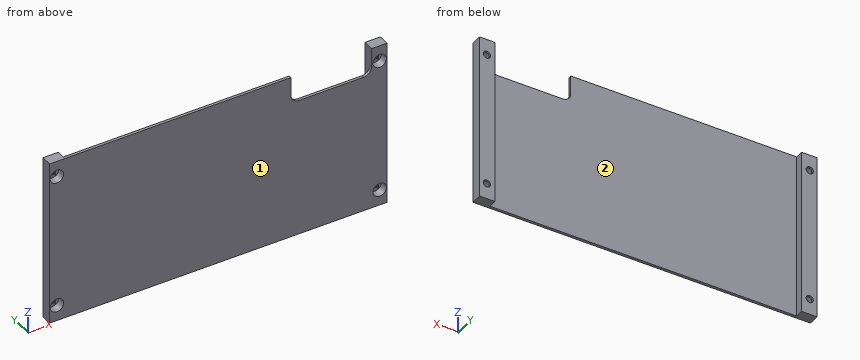
```python
from build123d import *

# Parameters (mm, degrees)
SKETCH1_W           = 126
SKETCH1_H           = 61.8
BOSS_EXTRUDE1_DEPTH = 1
SKETCH2_W           = 6
SKETCH2_H           = 61.8
BOSS_EXTRUDE2_DEPTH = 3
SKETCH3_R           = 1.35
CUT_EXTRUDE1_DEPTH  = 5
SKETCH4_R           = 2.5
CUT_EXTRUDE2_DEPTH  = 3
SKETCH5_W           = 30
SKETCH5_H           = 10
CUT_EXTRUDE3_DEPTH  = 5
FILLET1_R           = 3
CUT_EXTRUDE4_DEPTH  = 0.2
SKETCH7_W           = 2.7
SKETCH7_H           = 2.7
CUT_EXTRUDE5_DEPTH  = 0.2
SKETCH8_W           = 0.3
SKETCH8_H           = 61.8
CUT_EXTRUDE6_DEPTH  = 5


with BuildPart() as part:
    # Sketch1 → Boss-Extrude1 (new body)
    with BuildSketch(Plane(origin=(0, 0, 0), x_dir=(1, 0, 0), z_dir=(0, 1, 0))):
        Rectangle(SKETCH1_W, SKETCH1_H)
    extrude(amount=BOSS_EXTRUDE1_DEPTH)

    # Sketch2 → Boss-Extrude2 (add)
    with BuildSketch(Plane(origin=(0, 1, 0), x_dir=(1, 0, 0), z_dir=(0, 1, 0))):
        with Locations((-60, 0)):
            Rectangle(SKETCH2_W, SKETCH2_H)
        with Locations((60, 0)):
            Rectangle(SKETCH2_W, SKETCH2_H)
    extrude(amount=BOSS_EXTRUDE2_DEPTH)

    # Sketch3 → Cut-Extrude1 (cut, through all)
    with BuildSketch(Plane(origin=(0, 4, 0), x_dir=(1, 0, 0), z_dir=(0, 1, 0))):
        with Locations((-60, 25)):
            Circle(SKETCH3_R)
        with Locations((-60, -25)):
            Circle(SKETCH3_R)
        with Locations((60, -25)):
            Circle(SKETCH3_R)
        with Locations((60, 25)):
            Circle(SKETCH3_R)
    extrude(amount=-CUT_EXTRUDE1_DEPTH, mode=Mode.SUBTRACT)

    # Sketch4 → Cut-Extrude2 (cut)
    with BuildSketch(Plane.XZ):
        with Locations((60, -25)):
            Circle(SKETCH4_R)
        with Locations((60, 25)):
            Circle(SKETCH4_R)
        with Locations((-60, 25)):
            Circle(SKETCH4_R)
        with Locations((-60, -25)):
            Circle(SKETCH4_R)
    extrude(amount=-CUT_EXTRUDE2_DEPTH, mode=Mode.SUBTRACT)

    # Sketch5 → Cut-Extrude3 (cut, through all)
    with BuildSketch(Plane.XZ):
        with Locations((42, 25.9)):
            Rectangle(SKETCH5_W, SKETCH5_H)
    extrude(amount=-CUT_EXTRUDE3_DEPTH, mode=Mode.SUBTRACT)

    # Fillet1
    fillet1_edges = [part.edges().sort_by_distance(p)[0] for p in [
        (27, 0.5, 20.9),
        (57, 0.5, 20.9),
    ]]
    fillet(fillet1_edges, radius=FILLET1_R)

    # Sketch6 → Cut-Extrude4 (cut)
    with BuildSketch(Plane.XZ.offset(-3)):
        with BuildLine():
            Line((-61.35, 22.895837459), (-61.35, 27.104162541))
            ThreePointArc((-61.35, 27.104162541), (-60, 27.5), (-58.65, 27.104162541))
            Line((-58.65, 27.104162541), (-58.65, 22.895837459))
            ThreePointArc((-58.65, 22.895837459), (-60, 22.5), (-61.35, 22.895837459))
        make_face()
        with BuildLine():
            Line((-61.35, -27.104162541), (-61.35, -22.895837459))
            ThreePointArc((-61.35, -22.895837459), (-60, -22.5), (-58.65, -22.895837459))
            Line((-58.65, -22.895837459), (-58.65, -27.104162541))
            ThreePointArc((-58.65, -27.104162541), (-60, -27.5), (-61.35, -27.104162541))
        make_face()
    cut_extrude4 = extrude(amount=-CUT_EXTRUDE4_DEPTH, mode=Mode.SUBTRACT)

    # Sketch7 → Cut-Extrude5 (cut)
    with BuildSketch(Plane.XZ.offset(-3.2)):
        with Locations((-60, -25)):
            Rectangle(SKETCH7_W, SKETCH7_H)
        with Locations((-60, 25)):
            Rectangle(SKETCH7_W, SKETCH7_H)
    cut_extrude5 = extrude(amount=-CUT_EXTRUDE5_DEPTH, mode=Mode.SUBTRACT)

    # Mirror1: Cut-Extrude4, Cut-Extrude5 across plane
    add(cut_extrude4.mirror(Plane(origin=(0, 0, 0), x_dir=(0, 0, 1), z_dir=(1, 0, 0))), mode=Mode.SUBTRACT)
    add(cut_extrude5.mirror(Plane(origin=(0, 0, 0), x_dir=(0, 0, 1), z_dir=(1, 0, 0))), mode=Mode.SUBTRACT)

    # Sketch8 → Cut-Extrude6 (cut, through all)
    with BuildSketch(Plane(origin=(0, 4, 0), x_dir=(1, 0, 0), z_dir=(0, 1, 0))):
        with Locations((-62.85, 0)):
            Rectangle(SKETCH8_W, SKETCH8_H)
        with Locations((62.85, 0)):
            Rectangle(SKETCH8_W, SKETCH8_H)
    extrude(amount=-CUT_EXTRUDE6_DEPTH, mode=Mode.SUBTRACT)


solid = part.part
```
Can you work these out from the model? Positions are in its coordinate system, mm. Face numbers are marked on the shaded views. A direction names the side the tool comes from. Round coordinates to 2 decimals unless told otherwise and drop trailing zeros. Order: outer loops, then holes, each group sorted by start corner. A loop starts at its lowest first (then second) coordinate and runs counter-clockwise, first axis right, second up.
(1) If we section it at A-A (y = 2): Please give me the cut outline in (x, z).
Results are:
outline: (-62.7, -30.9) - (-57, -30.9) - (-57, 30.9) - (-62.7, 30.9) - close; (57, -30.9) - (62.7, -30.9) - (62.7, 30.9) - (57, 30.9) - close; hole circle Ø5 at (-60, -25); hole circle Ø5 at (-60, 25); hole circle Ø5 at (60, -25); hole circle Ø5 at (60, 25)
(2) If we section it at B-B (z = 12): Please give me the cut outline in (x, y).
Results are:
outline: (-62.7, 0) - (62.7, 0) - (62.7, 4) - (57, 4) - (57, 1) - (-57, 1) - (-57, 4) - (-62.7, 4) - close
(3) On a 3-axis mill with a long thin cutter (end or side, diameter ignored), from which of +Z, -Z, +X, -X, +Y, -Y can I reach the whole of each face in a straight line? I mean the marked faces 1 and 2. Say none if no direction works.
Results are:
face 1: +Z, -Z, +X, -X, -Y
face 2: +Z, -Z, +Y
(4) If I drill on L1, parallel to Z at x = -60, y = 1.3; L2, parallel to Z at x = 60, y = 3.75; L3, parallel to X at y = 1.45, z = 25, over which ranges is the centre line in solid material (lowest first)?
Results are:
L1: z = -30.9 to -27.5, -22.5 to 22.5, 27.5 to 30.9
L2: z = -30.9 to -26.35, -23.65 to 23.65, 26.35 to 30.9
L3: x = -62.7 to -62.5, -57.5 to -57, 57 to 57.5, 62.5 to 62.7
(5) I'm going to push flat-ended pins straight in: pin 1 (1.5 mm diameter, centred on x = -59, z = -25.5, fed in from -Y); pin 2 (1.5 mm diameter, centred on x = 20.5, z = 21, fed in from +Y); pin 3 (0.5 mm diameter, centred on x = 42.5, y = 0.5, fed in from +Z). Where does each tip first touch, or does it pass through?
Results are:
pin 1: stops at y = 3
pin 2: stops at y = 1
pin 3: stops at z = 20.9
(6) If we section it at D-D (x = -36): Please give me the cut outline in (y, z).
Results are:
outline: (0, -30.9) - (1, -30.9) - (1, 30.9) - (0, 30.9) - close
(7) If we section it at C-C (x = 49.5): Please give me the cut outline in (y, z), plus the area to 3 significant figures.
Results are:
outline: (0, -30.9) - (1, -30.9) - (1, 20.9) - (0, 20.9) - close
area: 51.8 mm2
